```python
from build123d import *

# Parameters (mm, degrees)
SKETCH1_R           = 2.6
BOSS_EXTRUDE1_DEPTH = 10
SKETCH2_R           = 2.6
CUT_EXTRUDE1_DEPTH  = 8


with BuildPart() as part:
    # Sketch1 → Boss-Extrude1 (new body)
    with BuildSketch(Plane.XY):
        with BuildLine():
            Line((0, 0), (0, 19))
            Line((0, 19), (130, 19))
            Line((130, 19), (130, 0))
            Line((130, 0), (120.963869458, 0))
            ThreePointArc((120.963869458, 0), (120.092881118, 0.508696316), (120.108029897, 1.517241379))
            ThreePointArc((120.108029897, 1.517241379), (116, 8.8), (111.891970103, 1.517241379))
            ThreePointArc((111.891970103, 1.517241379), (111.907118882, 0.508696316), (111.036130542, 0))
            Line((111.036130542, 0), (108.963869458, 0))
            ThreePointArc((108.963869458, 0), (108.092881118, 0.508696316), (108.108029897, 1.517241379))
            ThreePointArc((108.108029897, 1.517241379), (104, 8.8), (99.891970103, 1.517241379))
            ThreePointArc((99.891970103, 1.517241379), (99.907118882, 0.508696316), (99.036130542, 0))
            Line((99.036130542, 0), (96.963869458, 0))
            ThreePointArc((96.963869458, 0), (96.092881118, 0.508696316), (96.108029897, 1.517241379))
            ThreePointArc((96.108029897, 1.517241379), (92, 8.8), (87.891970103, 1.517241379))
            ThreePointArc((87.891970103, 1.517241379), (87.907118882, 0.508696316), (87.036130542, 0))
            Line((87.036130542, 0), (84.963869458, 0))
            ThreePointArc((84.963869458, 0), (84.092881118, 0.508696316), (84.108029897, 1.517241379))
            ThreePointArc((84.108029897, 1.517241379), (80, 8.8), (75.891970103, 1.517241379))
            ThreePointArc((75.891970103, 1.517241379), (75.907118882, 0.508696316), (75.036130542, 0))
            Line((75.036130542, 0), (54.963869458, 0))
            ThreePointArc((54.963869458, 0), (54.092881118, 0.508696316), (54.108029897, 1.517241379))
            ThreePointArc((54.108029897, 1.517241379), (50, 8.8), (45.891970103, 1.517241379))
            ThreePointArc((45.891970103, 1.517241379), (45.907118882, 0.508696316), (45.036130542, 0))
            Line((45.036130542, 0), (42.963869458, 0))
            ThreePointArc((42.963869458, 0), (42.092881118, 0.508696316), (42.108029897, 1.517241379))
            ThreePointArc((42.108029897, 1.517241379), (38, 8.8), (33.891970103, 1.517241379))
            ThreePointArc((33.891970103, 1.517241379), (33.907118882, 0.508696316), (33.036130542, 0))
            Line((33.036130542, 0), (30.963869458, 0))
            ThreePointArc((30.963869458, 0), (30.092881118, 0.508696316), (30.108029897, 1.517241379))
            ThreePointArc((30.108029897, 1.517241379), (26, 8.8), (21.891970103, 1.517241379))
            ThreePointArc((21.891970103, 1.517241379), (21.907118882, 0.508696316), (21.036130542, 0))
            Line((21.036130542, 0), (18.963869458, 0))
            ThreePointArc((18.963869458, 0), (18.092881118, 0.508696316), (18.108029897, 1.517241379))
            ThreePointArc((18.108029897, 1.517241379), (14, 8.8), (9.891970103, 1.517241379))
            ThreePointArc((9.891970103, 1.517241379), (9.907118882, 0.508696316), (9.036130542, 0))
            Line((9.036130542, 0), (0, 0))
        make_face()
        with Locations((5, 14)):
            Circle(SKETCH1_R, mode=Mode.SUBTRACT)
        with Locations((65, 14)):
            Circle(SKETCH1_R, mode=Mode.SUBTRACT)
        with Locations((125, 14)):
            Circle(SKETCH1_R, mode=Mode.SUBTRACT)
    extrude(amount=BOSS_EXTRUDE1_DEPTH)

    # Sketch2 → Cut-Extrude1 (cut)
    with BuildSketch(Plane.XZ):
        with Locations((4.6, 5)):
            Circle(SKETCH2_R)
        with Locations((65, 5)):
            Circle(SKETCH2_R)
        with Locations((125.4, 5)):
            Circle(SKETCH2_R)
    extrude(amount=-CUT_EXTRUDE1_DEPTH, mode=Mode.SUBTRACT)


solid = part.part
```
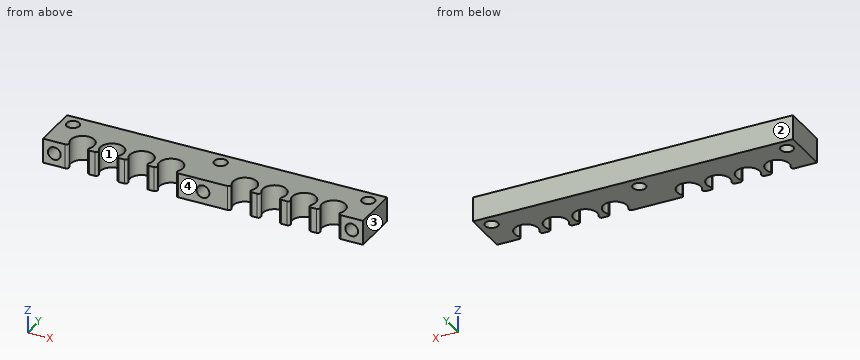
Verification items for the finished model (mm, model axes). Face numbers are marked on the shaded views. Coordinates: 2 decimals unless noted, no trailing zeros. Loops run counter-clockwise (first coordinate to the right, second up) from the corner with the lowest first, then second, coordinate; pieces in that order, holes last. Notation, with made-up numbers: (-38, -6) -> (-14, -6) arc R19 ccw to (-14, 12) -> close; hole circle Ø3 at (42, 62.25). An arc over 180 degrees is marked (long way). Answer in a Markdown table with one row per item.
1) Scan lines: line 1 along X through (y, z) = (16, 8.75); line 2 along Z through (x, y) = (4.6, 3.75); line 3 along Y through (x, z) = (5, 3.25). Record each from-to range of solid material in increasing order. Write a range as from..to.
The answers:
| item | result |
|---|---|
| line 1 | x = 0..3.34, 6.66..63.34, 66.66..123.34, 126.66..130 |
| line 2 | z = 0..2.4, 7.6..10 |
| line 3 | y = 8..11.4, 16.6..19 |
2) Section check C-C (x = 4.6). Record the cut outline in (y, z).
The answers:
| item | result |
|---|---|
| outline | (0, 0) -> (11.43, 0) -> (11.43, 10) -> (0, 10) -> (0, 7.6) -> (8, 7.6) -> (8, 2.4) -> (0, 2.4) -> close; (16.57, 0) -> (19, 0) -> (19, 10) -> (16.57, 10) -> close |
3) Section check B-B (y = 4). Give the number of separate pieces and of enclosed holes in the cut face, and give its area (3 significant figures).
The answers:
| item | result |
|---|---|
| separate pieces | 9 |
| enclosed holes | 3 |
| area | 468 mm2 |
4) Draft check along Y on the marked faces 1, 2, 3 and 4. Enter one of: released by +Y, released by -Y, zero draft, split by the parting line, or undercut.
The answers:
| item | result |
|---|---|
| face 1 | undercut |
| face 2 | released by +Y |
| face 3 | zero draft |
| face 4 | released by -Y |
5) Depth check by flat-ended pin: P1, Ø1.6, axis at x = 4, z = 5.5, coming from the -Y side; P2, Ø2, axis at x = 113.5, z = 7, coming from the -Y side. Enter the tip coordinate at first touch or a pass-through.
The answers:
| item | result |
|---|---|
| P1 | stops at y = 8 |
| P2 | stops at y = 7.28 |
6) Section check A-A (x = 65). Record the cut outline in (y, z), and give its area (3 significant figures).
The answers:
| item | result |
|---|---|
| outline | (0, 0) -> (11.4, 0) -> (11.4, 10) -> (0, 10) -> (0, 7.6) -> (8, 7.6) -> (8, 2.4) -> (0, 2.4) -> close; (16.6, 0) -> (19, 0) -> (19, 10) -> (16.6, 10) -> close |
| area | 96.4 mm2 |
